from build123d import *

# Parameters (mm, degrees)
SKETCH1_W           = 125
SKETCH1_H           = 125
BOSS_EXTRUDE1_DEPTH = 6
FILLET1_R           = 10
SKETCH9_R           = 3
CUT_EXTRUDE1_DEPTH  = 10


with BuildPart() as part:
    # Sketch1 → Boss-Extrude1 (new body)
    with BuildSketch(Plane.XY):
        Rectangle(SKETCH1_W, SKETCH1_H)
    extrude(amount=BOSS_EXTRUDE1_DEPTH)

    # Fillet1
    fillet1_edges = [part.edges().sort_by_distance(p)[0] for p in [
        (-62.5, 62.5, 3),
        (62.5, 62.5, 3),
        (62.5, -62.5, 3),
        (-62.5, -62.5, 3),
    ]]
    fillet(fillet1_edges, radius=FILLET1_R)

    # Sketch9 → Cut-Extrude1 (cut)
    with BuildSketch(Plane.XY.offset(6)):
        with Locations((50.3, 30)):
            Circle(SKETCH9_R)
        with Locations((50.3, -30)):
            Circle(SKETCH9_R)
        with Locations((-50.3, 30)):
            Circle(SKETCH9_R)
        with Locations((-50.3, -30)):
            Circle(SKETCH9_R)
    extrude(amount=-CUT_EXTRUDE1_DEPTH, mode=Mode.SUBTRACT)


solid = part.part
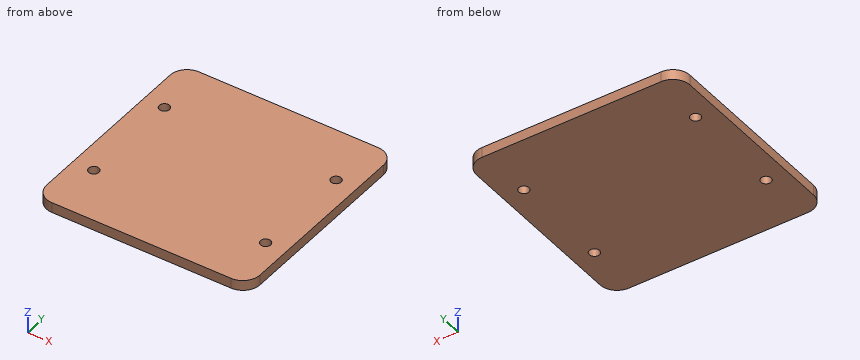
CAD build for the part. Positions are in the model's coordinates, mm. Coordinates: 2 decimals unless noted, no trailing zeros. Write each loop counter-clockwise with the first axis right and the second up, starting at its lowest first coordinate (ties: lowest second). Pieces come first, ordered by that corner, then holes. Notation, with made-up numbers: M 17.5,75 L 40.5,75 A18 cw 40.5,92 Z; hole C 39.25,14 d3. An arc over 180 degrees is marked long. Return JSON: item names as keys, results as strings.
Item 1: Slice it at A-A, the plane y = 30. Write the cut outline in (x, z).
Findings below:
{"outline": "M -62.5,0 L -53.3,0 L -53.3,6 L -62.5,6 Z; M -47.3,0 L 47.3,0 L 47.3,6 L -47.3,6 Z; M 53.3,0 L 62.5,0 L 62.5,6 L 53.3,6 Z"}
Item 2: Slice it at B-B, the plane x = -50.3. Write the cut outline in (y, z), and give its area (3 significant figures).
Findings below:
{"outline": "M -62.5,0 L -33,0 L -33,6 L -62.5,6 Z; M -27,0 L 27,0 L 27,6 L -27,6 Z; M 33,0 L 62.5,0 L 62.5,6 L 33,6 Z", "area": "678 mm2"}
Item 3: Probe line 1 (Y direction, x = 50.3, z = 3.75); line 2 (X direction, y = 29, z = 4.2); line 3 (X direction, y = -53, z = 5.1). List the from-to ranges inside material, lowest first. Write a range as from..to.
Findings below:
{"line 1": "y = -62.5..-33, -27..27, 33..62.5", "line 2": "x = -62.5..-53.13, -47.47..47.47, 53.13..62.5", "line 3": "x = -62.49..62.49"}
